from build123d import *

# Parameters (mm, degrees)
SALIENTE_EXTRUIR1_DEPTH = 25
CROQUIS2_R              = 3.2
CORTAR_EXTRUIR1_DEPTH   = 12
REDONDEO1_R             = 2


with BuildPart() as part:
    # Croquis1 → Saliente-Extruir1 (new body)
    with BuildSketch(Plane(origin=(0, 0, 0), x_dir=(1, 0, 0), z_dir=(0, 1, 0))):
        with BuildLine():
            Line((-4.858898944, 1.179449472), (-10, -20))
            Line((-10, -20), (10, -20))
            Line((10, -20), (4.858898944, 1.179449472))
            ThreePointArc((4.858898944, 1.179449472), (0, 5), (-4.858898944, 1.179449472))
        make_face()
    extrude(amount=SALIENTE_EXTRUIR1_DEPTH)

    # Croquis2 → Cortar-Extruir1 (cut)
    with BuildSketch(Plane.XY.offset(20)):
        with Locations((0, 7.8)):
            Circle(CROQUIS2_R)
    extrude(amount=-CORTAR_EXTRUIR1_DEPTH, mode=Mode.SUBTRACT)

    # Redondeo1
    redondeo1_edges = [part.edges().sort_by_distance(p)[0] for p in [
        (10, 12.5, 20),
        (-10, 12.5, 20),
    ]]
    fillet(redondeo1_edges, radius=REDONDEO1_R)


solid = part.part
Input: part model. Units: mm. Frame: model coordinates. Round coordinates to 2 decimals unless told otherwise and drop trailing zeros. Order: outer loops, then holes, each group sorted by start corner. A loop starts at its lowest first (then second) coordinate and runs counter-clockwise, first axis right, second up. Notation, with made-up numbers: (82, 24) - (112, 24) arc R31 ccw to (112, 49) - close; hole circle Ø6 at (71.25, 78). An arc over 180 degrees is marked (long way). Answer as a JSON object with one key per item and string values. Group by question number.
(1) Draft query along Y for faces 1 (the face through (0, 0, 10)), 2 (the face through (-0.694, 4.676, 14.084)), 3 (the face through (0, 8, 8)), 4 (the face through (0, 12, 20)). Return one class per face: released by +Y, released by -Y, zero draft, split by the parting line, or undercut.
(2) Material intervals for probe 1 along Y at (x, z) = (0, 17); probe 2 along X at (y, z) = (18.75, 9.5); probe 3 along Z at (x, y) = (3.5, 19.5), sorted ascending. Write a range as from..to.
(3) Pin query (flat end, axial travel): P1, Ø12, axis at y = 14, z = 17.5, coming from the -X side; P2, Ø8, axis at y = 12, z = 5.5, coming from the +X side; P3, Ø2, axis at y = 7, z = 7.5, coming from the -X side; P4, Ø8, axis at y = 9.5, z = 7.5, coming from the +X side. Return the tip coordinate at first contact, or that it passes through.
(4) Cut plane D-D (y = 14.75). Return loops of the section in (x, z).
(5) Cut plane B-B (z = 14.5). Return loops of the section in (x, y).
(6) Cut plane C-C (x = 0). Return loops of the section in (y, z), then the cut area to 3 significant figures.
(7) Cut plane A-A (y = 7.8). Return loops of the section in (x, z).
Here are the results:
{
 "1": {"face 1": "released by -Y", "face 2": "undercut", "face 3": "undercut", "face 4": "zero draft"},
 "2": {"probe 1": "y = 0..4.6, 11..25", "probe 2": "x = -7.45..7.45", "probe 3": "z = -3.57..20"},
 "3": {"P1": "stops at x = -9.46", "P2": "stops at x = 7.45", "P3": "stops at x = -7.21", "P4": "stops at x = 7.94"},
 "4": {"outline": "(-9.4, 17.53) - (-4.86, -1.18) arc R5 ccw to (4.86, -1.18) - (9.4, 17.53) arc R2 ccw to (7.46, 20) - (-7.46, 20) arc R2 ccw to start"},
 "5": {"outline": "(-8.66, 0) - (8.66, 0) - (8.66, 25) - (-8.66, 25) - close; hole circle Ø6.4 at (0, 7.8)"},
 "6": {"outline": "(0, -5) - (25, -5) - (25, 20) - (11, 20) - (11, 8) - (4.6, 8) - (4.6, 20) - (0, 20) - close", "area": "548 mm^2"},
 "7": {"outline": "(-9.4, 17.53) - (-4.86, -1.18) arc R5 ccw to (4.86, -1.18) - (9.4, 17.53) arc R2 ccw to (7.46, 20) - (3.2, 20) - (3.2, 8) - (-3.2, 8) - (-3.2, 20) - (-7.46, 20) arc R2 ccw to start"}
}
